from build123d import *

# Parameters (mm, degrees)
SKETCH1_R           = 3.295
BOSS_EXTRUDE1_DEPTH = 5


with BuildPart() as part:
    # Sketch1 → Boss-Extrude1 (new body)
    with BuildSketch(Plane(origin=(0, 0, 0), x_dir=(1, 0, 0), z_dir=(0, 1, 0))):
        Polygon((0, 0), (0, 70), (25.54, 70), (50.9, 45.2), (50.9, 0), align=None)
        with Locations((14.667483235, 62.445)):
            Circle(SKETCH1_R, mode=Mode.SUBTRACT)
        with Locations((33.008944764, 44.743844982)):
            Circle(SKETCH1_R, mode=Mode.SUBTRACT)
        with Locations((12.695, 12.995)):
            Circle(SKETCH1_R, mode=Mode.SUBTRACT)
        with Locations((38.135, 12.995)):
            Circle(SKETCH1_R, mode=Mode.SUBTRACT)
        with Locations((16, 51.333944626)):
            Circle(SKETCH1_R, mode=Mode.SUBTRACT)
        with Locations((27, 32.281385742)):
            Circle(SKETCH1_R, mode=Mode.SUBTRACT)
    extrude(amount=BOSS_EXTRUDE1_DEPTH)


solid = part.part
Build history of the part. All positions in model axes, mm. Coordinates: 2 decimals unless noted, no trailing zeros. Order: outer loops, then holes, each group sorted by start corner. A loop starts at its lowest first (then second) coordinate and runs counter-clockwise, first axis right, second up. Notation, with made-up numbers: M 32,80 L 50,80 A15 cw 50,96 Z; hole C -13.75,53.25 d5. An arc over 180 degrees is marked long. One line per question, with ' | ' between items. Start each with the question number.
Q1. Flat gauge pin, fed straight in: pin 1 Ø7.5 at (x, z) = (33.01, -44.74) entering from +Y. Where does the tip first touch, or does it go through?
Q2. Probe L1, parallel to Z at x = 14, y = 2.95; L2, parallel to Z at x = 38, y = 1.9; L3, parallel to Z at x = 28, y = 1.6. List the from-to ranges inside material, lowest first. Write a range as from..to.
Q3. Saw through at B-B (x = 27). List the corners of the cut face in (y, z).
Q4. Saw through at C-C (y = 3.9). List the corners of the cut face in (x, z) (3 decimals).
Q5. Two-plate mould, pull along X, no slides. Class faces 1 (the face through (50.9, 2, -23)), 2 (the face through (20, 0, -35)), 3 (the face through (37.42, 2.46, -9.78)), 4 (the face through (30.58, 2.46, -46.97)): +X half, -X half, draft (parallel to the pull), parting line (faces both ways), or undercut.
Q6. Saw through at D-D (z = -55.5). List the corners of the cut face in (x, y).
Q7. Saw through at A-A (z = -46.5). List the corners of the cut face in (x, y), then the cut area to 3 significant figures.
Check values:
1) pin 1: stops at y = 5
2) L1: z = -70..-65.67, -59.22..-53.95, -48.72..-16.02, -9.97..0 | L2: z = -57.82..-16.29, -9.7..0 | L3: z = -67.59..-35.42, -29.14..0
3) outline: M 0,-68.57 L 5,-68.57 L 5,-35.58 L 0,-35.58 Z; M 0,-28.99 L 5,-28.99 L 5,0 L 0,0 Z
4) outline: M 0,-70 L 25.54,-70 L 50.9,-45.2 L 50.9,0 L 0,0 Z; hole C 12.695,-12.995 d6.59; hole C 14.667,-62.445 d6.59; hole C 16,-51.334 d6.59; hole C 27,-32.281 d6.59; hole C 33.009,-44.744 d6.59; hole C 38.135,-12.995 d6.59
5) face 1: +X half | face 2: draft | face 3: undercut | face 4: undercut
6) outline: M 0,0 L 40.37,0 L 40.37,5 L 0,5 Z
7) outline: M 0,0 L 30.22,0 L 30.22,5 L 0,5 Z; M 35.8,0 L 49.57,0 L 49.57,5 L 35.8,5 Z | area: 220 mm2
